Design review of the part built by this model. Coordinates are the model's own, in mm. A direction names the side the tool comes from. Round coordinates to 2 decimals unless told otherwise and drop trailing zeros. Order: outer loops, then holes, each group sorted by start corner. A loop starts at its lowest first (then second) coordinate and runs counter-clockwise, first axis right, second up. Notation, with made-up numbers: (-39.75, 21.25) - (15.25, 21.25) arc R19 cw to (15.25, 47.25) - close; hole circle Ø9 at (-25.5, 52.5). An arc over 180 degrees is marked (long way). Use CSV: the item, a comma, the result in double quotes.
from build123d import *

# Parameters (mm, degrees)
SALIENTE_EXTRUIR3_DEPTH = 250
CROQUIS6_R              = 10
CORTAR_EXTRUIR1_DEPTH   = 264
CROQUIS7_W              = 200
CROQUIS7_H              = 165
CORTAR_EXTRUIR3_DEPTH   = 264


with BuildPart() as part:
    # Croquis3 → Saliente-Extruir3 (new body)
    with BuildSketch(Plane.XY):
        with BuildLine():
            Line((200, 150), (67.909088668, 278.654541869))
            ThreePointArc((67.909088668, 278.654541869), (24.449494329, 286.853517788), (0, 250))
            Line((0, 250), (0, 150))
            Line((0, 150), (0, 0))
            Line((0, 0), (200, 0))
            Line((200, 0), (200, 150))
        make_face()
    extrude(amount=SALIENTE_EXTRUIR3_DEPTH)

    # Croquis6 → Cortar-Extruir1 (cut)
    with BuildSketch(Plane(origin=(0, 0, 0), x_dir=(-1, 0, 0), z_dir=(0, 0, -1))):
        with Locations((-40, 250)):
            Circle(CROQUIS6_R)
    extrude(amount=-CORTAR_EXTRUIR1_DEPTH, mode=Mode.SUBTRACT)

    # Croquis7 → Cortar-Extruir3 (cut)
    with BuildSketch(Plane.ZY):
        with Locations((125, 207.5)):
            Rectangle(CROQUIS7_W, CROQUIS7_H)
    extrude(amount=-CORTAR_EXTRUIR3_DEPTH, mode=Mode.SUBTRACT)


solid = part.part
1) We need section C-C (x = 143). Give the boundary of the cut face in (y, z), then the cut area to 3 significant figures.
Data:
outline,"(0, 0) - (205.52, 0) - (205.52, 25) - (125, 25) - (125, 225) - (205.52, 225) - (205.52, 250) - (0, 250) - close"
area,"35,300 mm2"
2) To check wall thickness, follow L1, parallel to Y at x = 40, z = 232.75; L2, parallel to Z at x = 28.5, y = 218; L3, parallel to Y at x = 58.5, z = 185. State the ranges of each line that lie inside material, in increasing order. Write a range as from..to.
Data:
L1,"y = 0..240, 260..290"
L2,"z = 0..25, 225..250"
L3,"y = 0..125"
3) Insertion check: pin 1 Ø1 at (x, z) = (165, 111.5) entering from +Y. The pin has a flat end and moves straight along its axis. Give the tip position at first contact, or say it passes through.
Data:
pin 1,"stops at y = 125"
4) We need section D-D (z = 89). Give the boundary of the cut face in (x, y).
Data:
outline,"(0, 0) - (200, 0) - (200, 125) - (0, 125) - close"
5) We need section B-B (z = 18). Give the boundary of the cut face in (x, y).
Data:
outline,"(0, 0) - (200, 0) - (200, 150) - (67.91, 278.65) arc R40 ccw to (0, 250) - close; hole circle Ø20 at (40, 250)"
6) We need section A-A (x = 40). Give the boundary of the cut face in (y, z).
Data:
outline,"(0, 0) - (240, 0) - (240, 25) - (125, 25) - (125, 225) - (240, 225) - (240, 250) - (0, 250) - close; (260, 0) - (290, 0) - (290, 25) - (260, 25) - close; (260, 225) - (290, 225) - (290, 250) - (260, 250) - close"
7) For faces 1 (the face through (0, 71, 123)), 2 (the face through (76, 188, 25)), list the 3-axis set-ups (+Z, -Z, +X, -X, +Y, -Y) from which the entire face can be reached by the end or side of a thin tool; tool diameter is ignored.
Data:
face 1,"+Z, -Z, -X, +Y, -Y"
face 2,"+X, -X, +Y"
8) The part is to be moulded in two halves that separate along X. For faces 3 (the face through (134.879, 213.427, 12.325)), 4 (the face through (99, 115, 0)), 5 (the face through (41.302, 259.915, 12.325)), say which applies: +X half, -X half, draft (parallel to the pull), parting line (faces both ways), or undercut.
Data:
face 3,"+X half"
face 4,"draft"
face 5,"undercut"
